Model file for the job. Use its own axes, mm. A direction names the side the tool comes from. Give positions to 0.01 mm unless a question says otherwise; leave off trailing zeros. Order: outer loops, then holes, each group sorted by start corner. A loop starts at its lowest first (then second) coordinate and runs counter-clockwise, first axis right, second up. Notation, with made-up numbers: (-18, 14.5) -> (28, 14.5) arc R27 cw to (28, 38.5) -> close; hole circle Ø2 at (28, -24.5). An arc over 180 degrees is marked (long way). Answer in a Markdown table with one row per item. Add a question column.
Autodesk Inventor part; units mm, degrees
ref_plane "YZ Plane" through (0, 0, 0) normal (1, 0, 0) x (0, 1, 0)
ref_plane "XZ Plane" through (0, 0, 0) normal (0, 1, 0) x (-1, 0, 0)
ref_plane "XY Plane" through (0, 0, 0) normal (0, 0, 1) x (1, 0, 0)
sketch "Sketch1" plane through (0, 0, 0) normal (0, 1, 0) x (-1, 0, 0)
  line L0 (17.5, 14.325) -> (17.5, -14.325)
  line L1 (14.325, -17.5) -> (-14.325, -17.5)
  line L2 (-17.5, -14.325) -> (-17.5, 14.325)
  line L3 (-14.325, 17.5) -> (-13.175, 17.5)
  line L4 (-10, 20.675) -> (-10, 60)
  line L5 (-10, 60) -> (10, 60)
  line L6 (10, 60) -> (10, 20.675)
  line L7 (13.175, 17.5) -> (14.325, 17.5)
  arc A0 (10, 20.675) -> (13.175, 17.5) centre (13.175, 20.675) ccw
  arc A1 (-13.175, 17.5) -> (-10, 20.675) centre (-13.175, 20.675) ccw
  arc A2 (17.5, 14.325) -> (14.325, 17.5) centre (14.325, 14.325) ccw
  arc A3 (14.325, -17.5) -> (17.5, -14.325) centre (14.325, -14.325) ccw
  arc A4 (-17.5, -14.325) -> (-14.325, -17.5) centre (-14.325, -14.325) ccw
  arc A5 (-14.325, 17.5) -> (-17.5, 14.325) centre (-14.325, 14.325) ccw
  point P0 (0, 0)
  point P1 (17.5, 17.5)
  point P2 (17.5, -17.5)
  point P3 (-17.5, -17.5)
  point P4 (-17.5, 17.5)
  point P5 (-10, 17.5)
  point P6 (10, 17.5)
  point P7 (17.5, 0)
  point P8 (0, -17.5)
  point P9 (0, 60)
  dimension "d0" = 35
  dimension "d1" = 35
  dimension "d2" = 20
  dimension "d3" = 60
  dimension "d26" = 3.175
  dimension "d27" = 3.175
extrude "Extrusion1" add sketch "Sketch1" along normal blind 5.334
sketch "Sketch3" plane through (0, 5.334, 0) normal (0, 1, 0) x (1, 0, 0)
  point P0 (0, 0)
  point P1 (0, 0)
hole "Hole2" at (0, 5.334, 0) direction (0, -1, 0) diameter 16 end through all
sketch "Sketch6" plane through (10, 0, 60) normal (1, 0, 0) x (0, 0, -1)
  line L0 (0, 5.334) -> (39.325, 5.334)
  line L1 (0, 0) -> (39.325, 0)
  line L2 (14, 5.334) -> (8, 5.334)
  line L3 (8, 5.334) -> (8, 0)
  line L4 (8, 0) -> (14, 0)
  line L5 (14, 0) -> (14, 5.334)
  line L6 (0, 0) -> (0, 5.334)
  point P0 (60, 0)
  dimension "d41" = 6
  dimension "d42" = 8
extrude "Extrusion3" cut sketch "Sketch6" against normal blind 5.334 contours L0 L5 L1 L3
sketch "Sketch5" plane through (-10, 0, 60) normal (0, 0, 1) x (1, 0, 0)
  line L0 (0, 5.334) -> (20, 5.334)
  line L1 (0, 0) -> (6, 0)
  line L2 (6, 0) -> (6, 5.334)
  line L3 (6, 5.334) -> (0, 5.334)
  line L4 (0, 5.334) -> (0, 0)
  line L5 (20, 0) -> (14, 0)
  line L6 (14, 0) -> (14, 5.334)
  line L7 (14, 5.334) -> (20, 5.334)
  line L8 (20, 5.334) -> (20, 0)
  line L9 (20, 0) -> (20, 5.334)
  point P0 (10, 0)
  point P1 (20, 2.667)
  dimension "d45" = 6
  dimension "d46" = 6
extrude "Extrusion2" add sketch "Sketch5" along normal blind 5.334
mirror "Mirror1" about plane through (0, 0, 0) normal (1, 0, 0) of "Extrusion3"
equation "\"d46\" = d45"
properties part number "pitch_support"
Item 1: Which spindle directions (+Z, -Z, +X, -X, +Y, -Y) get a long thin tool onto all of the face, cutting with end or side? Do faces 4 (the flat face through (0, 0, 15)), 5 (the cylindrical face through (-16.59, 2.63, -16.55)), 6 (the flat face through (-10, 3, 34)), 7 (the flat face through (7, 3, 46)), 8 (the flat face through (-4, 3, 63)). Say none if no direction does.
Item 2: Saw through at D-D on x = 6. List the corners of the cut face in (y, z).
Item 3: Saw through at C-C on y = 1.7. List the corners of the cut face in (x, z) (3 decimals).
Item 4: Two-plate mould, pull along Z, no slides. Class faces 1 (the flat face through (4, 3, 63)), 2 (the flat face through (0, 3, -17.5)), 3 (the cylindrical face through (7.81, 2.63, -1.73)): pulls with the +Z half, pulls with the -Z half, needs draft (parallel to the pull), parting line crosses it, or undercut.
Item 5: Pin check, flat tips, straight feed: pin 1 Ø0.6 at (x, y) = (13.5, 3.5) entering from +Z; pin 2 Ø2.5 at (y, z) = (3, 63) entering from +X; pin 3 Ø1.6 at (x, y) = (-1, 1.5) entering from +Z. Stop position of each tip, or through.
Item 6: Saw through at B-B on x = 0. List the corners of the cut face in (y, z), plus the area to 3 significant figures.
Item 7: Wall check: line 1 (Z direction, x = 0, y = 3.4); line 2 (X direction, y = 3.95, z = 0); line 3 (Z direction, x = -9.5, y = 1.1). Give the ranges that are in metal, low to high.
Item 8: Saw through at A-A on z = 0. List the corners of the cut face in (x, y).
Evaluation:
| question | item | result |
|---|---|---|
| 1 | face 4 | +Z, -Z, +X, -X, -Y |
| 1 | face 5 | -Z, -X, +Y, -Y |
| 1 | face 6 | +Z, -X, +Y, -Y |
| 1 | face 7 | +X, +Y, -Y |
| 1 | face 8 | +Z, +Y, -Y |
| 2 | outline | (0, -17.5) -> (5.33, -17.5) -> (5.33, -5.29) -> (0, -5.29) -> close; (0, 5.29) -> (5.33, 5.29) -> (5.33, 46) -> (0, 46) -> close; (0, 52) -> (5.33, 52) -> (5.33, 65.33) -> (0, 65.33) -> close |
| 3 | outline | (-17.5, -14.325) arc R3.175 ccw to (-14.325, -17.5) -> (14.325, -17.5) arc R3.175 ccw to (17.5, -14.325) -> (17.5, 14.325) arc R3.175 ccw to (14.325, 17.5) -> (13.175, 17.5) arc R3.175 cw to (10, 20.675) -> (10, 46) -> (4.666, 46) -> (4.666, 52) -> (10, 52) -> (10, 65.334) -> (4, 65.334) -> (4, 60) -> (-4, 60) -> (-4, 65.334) -> (-10, 65.334) -> (-10, 52) -> (-4.666, 52) -> (-4.666, 46) -> (-10, 46) -> (-10, 20.675) arc R3.175 cw to (-13.175, 17.5) -> (-14.325, 17.5) arc R3.175 ccw to (-17.5, 14.325) -> close; hole circle Ø16 at (0, 0) |
| 4 | face 1 | needs draft |
| 4 | face 2 | pulls with the -Z half |
| 4 | face 3 | undercut |
| 5 | pin 1 | stops at z = 17.5 |
| 5 | pin 2 | stops at x = 10 |
| 5 | pin 3 | stops at z = 60 |
| 6 | outline | (0, -17.5) -> (5.33, -17.5) -> (5.33, -8) -> (0, -8) -> close; (0, 8) -> (5.33, 8) -> (5.33, 60) -> (0, 60) -> close |
| 6 | area | 328 mm2 |
| 7 | line 1 | z = -17.5 to -8, 8 to 60 |
| 7 | line 2 | x = -17.5 to -8, 8 to 17.5 |
| 7 | line 3 | z = -17.5 to 46, 52 to 65.33 |
| 8 | outline | (-17.5, 0) -> (-8, 0) -> (-8, 5.33) -> (-17.5, 5.33) -> close; (8, 0) -> (17.5, 0) -> (17.5, 5.33) -> (8, 5.33) -> close |
